Read the model definition and answer for the solid it produces. Units are mm, in the model's axes. Face numbers are marked on the shaded views. A direction names the side the tool comes from. Coordinates: 2 decimals unless noted, no trailing zeros. Loops run counter-clockwise (first coordinate to the right, second up) from the corner with the lowest first, then second, coordinate; pieces in that order, holes last. Notation, with made-up numbers: M 14.25,89 L 60.25,89 A17 cw 60.25,102 Z; hole C -2.75,37 d1. An arc over 180 degrees is marked long. One line per item, written item: value. Start each with the question number.
1. Determine the mould class of the marked faces 1, 2 and 3 for opening direction X: +X half, -X half, draft (parallel to the pull), parting line (faces both ways), or undercut.
2. The part is cut by section C-C (x = 11.5). Write down the section's boundary in (y, z), then the cut area to 3 significant figures.
3. A flat-ended cylindrical pin translates along its axis: pin 1 (1.5 mm diameter, centred on x = -16.5, z = 24.5, fed in from +Y). Find the tip coordinate at first contact, or state that the pin passes through.
4. The part is cut by section B-B (y = -31). Write down the section's boundary in (x, z).
5. For the marked faces 4 and 5, determine the directions among +Z, -Z, +X, -X, +Y, -Y from which every point of the face is accessible in a straight line to the end or side of a thin tool.
6. The part is cut by section A-A (z = 47.5). Write down the section's boundary in (x, y), then the cut area to 3 significant figures.
7. Consider probe 1 along X at (y, z) = (-15.5, 32.5); probe 2 along Z at (x, y) = (14, -68.5). Determine where each line is inside the solid, lowest interval first.
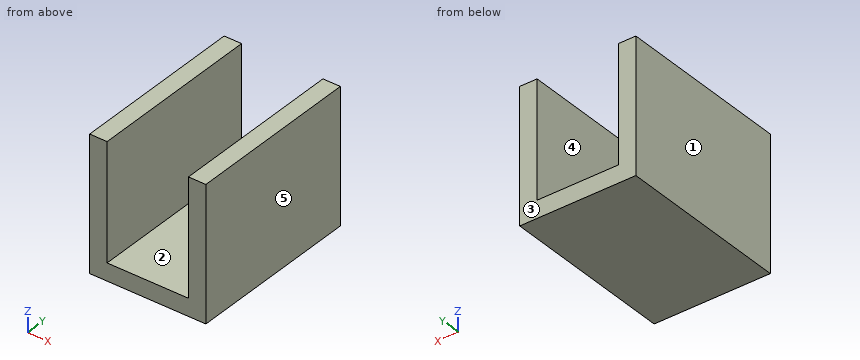
```python
from build123d import *

# Parameters (mm, degrees)
F0_W     = 7.62
F0_H     = 50.8
F1_DEPTH = 76.2


with BuildPart() as f1:
    # F0 (on Front) → F1 (new body)
    with BuildSketch(Plane.XZ):
        Polygon((0, 7.62), (0, 0), (25.4, 0), (25.4, 7.62), (17.78, 7.62), align=None)
        Polygon((-25.4, 0), (0, 0), (0, 7.62), (-17.78, 7.62), (-25.4, 7.62), align=None)
        with Locations((21.59, 33.02)):
            Rectangle(F0_W, F0_H)
        with Locations((-21.59, 33.02)):
            Rectangle(F0_W, F0_H)
    extrude(amount=F1_DEPTH)


solid = f1.part
```
Answer block:
1. face 1: -X half
1. face 2: undercut
1. face 3: draft
2. outline: M -76.2,0 L 0,0 L 0,7.62 L -76.2,7.62 Z
2. area: 581 mm2
3. pin 1: passes through
4. outline: M -25.4,0 L 25.4,0 L 25.4,58.42 L 17.78,58.42 L 17.78,7.62 L -17.78,7.62 L -17.78,58.42 L -25.4,58.42 Z
5. face 4: +Z, +Y, -Y
5. face 5: +Z, -Z, +X, +Y, -Y
6. outline: M -25.4,-76.2 L -17.78,-76.2 L -17.78,0 L -25.4,0 Z; M 17.78,-76.2 L 25.4,-76.2 L 25.4,0 L 17.78,0 Z
6. area: 1,160 mm2
7. probe 1: x = -25.4 to -17.78, 17.78 to 25.4
7. probe 2: z = 0 to 7.62
